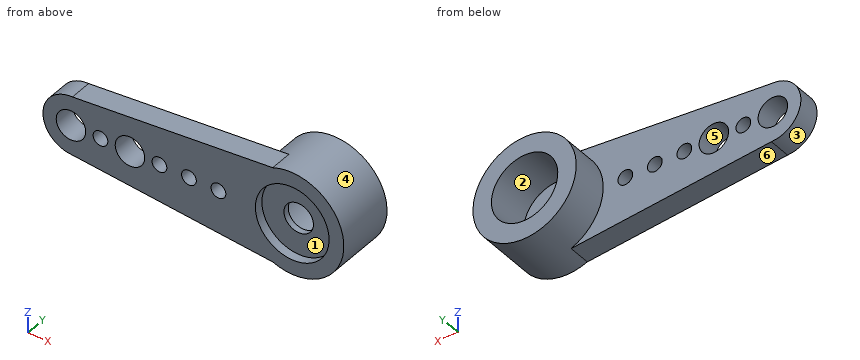
```python
from build123d import *

# Parameters (mm, degrees)
SKETCH1_R           = 3.5
BOSS_EXTRUDE1_DEPTH = 4
BOSS_EXTRUDE2_DEPTH = 1.5
SKETCH7_R           = 2.5
CUT_EXTRUDE4_DEPTH  = 0.6
SKETCH8_R           = 2.25
CUT_EXTRUDE5_DEPTH  = 3
SKETCH9_R           = 1
CUT_EXTRUDE6_DEPTH  = 18.590338257
SKETCH10_R          = 1
SKETCH10_R_2        = 0.5
CUT_EXTRUDE7_DEPTH  = 18.716094378


with BuildPart() as part:
    # Sketch1 → Boss-Extrude1 (new body)
    with BuildSketch(Plane(origin=(0, 0, 0), x_dir=(1, 0, 0), z_dir=(0, 1, 0))):
        with Locations(Location((0, 0, 0), (0, 0, 270))):
            Circle(SKETCH1_R)
    extrude(amount=BOSS_EXTRUDE1_DEPTH)

    # Sketch6 → Boss-Extrude2 (add)
    with BuildSketch(Plane.XZ):
        with BuildLine():
            Line((-14.9, 2), (-0.65, 3.301402389))
            Line((-0.65, 3.301402389), (0, 3.5))
            Line((0, 3.5), (0, -3.5))
            Line((0, -3.5), (-0.65, -3.301402389))
            Line((-0.65, -3.301402389), (-14.9, -2))
            ThreePointArc((-14.9, -2), (-16.9, 0), (-14.9, 2))
        make_face()
    extrude(amount=-BOSS_EXTRUDE2_DEPTH)

    # Sketch7 → Cut-Extrude4 (cut)
    with BuildSketch(Plane.XZ):
        with Locations(Location((0, 0, 0), (0, 0, 270))):
            Circle(SKETCH7_R)
    extrude(amount=-CUT_EXTRUDE4_DEPTH, mode=Mode.SUBTRACT)

    # Sketch8 → Cut-Extrude5 (cut)
    with BuildSketch(Plane(origin=(0, 4, 0), x_dir=(1, 0, 0), z_dir=(0, 1, 0))):
        with Locations(Location((0, 0, 0), (0, 0, 270))):
            Circle(SKETCH8_R)
    extrude(amount=-CUT_EXTRUDE5_DEPTH, mode=Mode.SUBTRACT)

    # Sketch9 → Cut-Extrude6 (cut, through all)
    with BuildSketch(Plane.XZ.offset(-0.6)):
        with Locations(Location((0, 0, 0), (0, 0, 270))):
            Circle(SKETCH9_R)
    extrude(amount=-CUT_EXTRUDE6_DEPTH, mode=Mode.SUBTRACT)

    # Sketch10 → Cut-Extrude7 (cut, through all)
    with BuildSketch(Plane.XZ):
        with Locations(Location((-15, 0, 0), (0, 0, 270))):
            Circle(SKETCH10_R)
        with Locations(Location((-13, 0, 0), (0, 0, 270))):
            Circle(SKETCH10_R_2)
        with Locations(Location((-11, 0, 0), (0, 0, 270))):
            Circle(SKETCH10_R)
        with Locations(Location((-9, 0, 0), (0, 0, 270))):
            Circle(SKETCH10_R_2)
        with Locations(Location((-7, 0, 0), (0, 0, 270))):
            Circle(SKETCH10_R_2)
        with Locations(Location((-5, 0, 0), (0, 0, 270))):
            Circle(SKETCH10_R_2)
    extrude(amount=-CUT_EXTRUDE7_DEPTH, mode=Mode.SUBTRACT)


solid = part.part
```
Here's how the part is built. I have some questions about the finished solid (model axes, mm). Face numbers are marked on the shaded views. A direction names the side the tool comes from. Give positions to 0.01 mm unless a question says otherwise; leave off trailing zeros. Write each loop counter-clockwise with the first axis right and the second up, starting at its lowest first coordinate (ties: lowest second). Pieces come first, ordered by that corner, then holes. Notation, with made-up numbers: (63.5, -19) -> (68.5, -19) arc R35 cw to (68.5, 14) -> close; hole circle Ø4 at (-39.5, -7). An arc over 180 degrees is marked (long way). Write each question's results on one line, items separated by ' | '.
Item 1: For pin 1 Ø1.5 at (x, y) = (-9.5, 1) entering from -Z; pin 2 Ø2 at (x, y) = (-2, 2.5) entering from +Z; pin 3 Ø2.5 at (x, z) = (0, 0) entering from +Y, each with a flat end and sliding along its axis, tell me the tip position at first contact or that it passes through.
Output:
pin 1: stops at z = -2.56 | pin 2: stops at z = 3.35 | pin 3: stops at y = 1
Item 2: Suppose I cut it at B-B on y = 1.3. Write out the boundary of the cut face in (x, z), plus the area to 3 significant figures.
Output:
outline: (-14.9, -2) -> (-1.32, -3.24) arc R3.5 ccw (long way) to (-1.32, 3.24) -> (-14.9, 2) arc R2 ccw to start; hole circle Ø2 at (-15, 0); hole circle Ø1 at (-13, 0); hole circle Ø2 at (-11, 0); hole circle Ø1 at (-9, 0); hole circle Ø1 at (-7, 0); hole circle Ø1 at (-5, 0); hole circle Ø4.5 at (0, 0) | area: 80.4 mm^2
Item 3: We'd pull the mould along X, two halves only. Please class the marked faces 4, 5 and 6: pulls with the +X half, pulls with the -X half, needs draft (parallel to the pull), parting line crosses it, or undercut.
Output:
face 4: parting line crosses it | face 5: undercut | face 6: pulls with the -X half
Item 4: Suppose I cut it at D-D on y = 3.75. Write out the boundary of the cut face in (x, z), plus the area to 3 significant figures.
Output:
outline: circle Ø7 at (0, 0); hole circle Ø4.5 at (0, 0) | area: 22.6 mm^2
Item 5: Suppose I cut it at C-C on z = 0.75. Write out the boundary of the cut face in (x, y).
Output:
outline: (-16.75, 0) -> (-15.66, 0) -> (-15.66, 1.5) -> (-16.75, 1.5) -> close; (-14.34, 0) -> (-11.66, 0) -> (-11.66, 1.5) -> (-14.34, 1.5) -> close; (-10.34, 0) -> (-2.38, 0) -> (-2.38, 0.6) -> (-0.66, 0.6) -> (-0.66, 1) -> (-2.12, 1) -> (-2.12, 4) -> (-3.42, 4) -> (-3.42, 1.5) -> (-10.34, 1.5) -> close; (0.66, 0.6) -> (2.38, 0.6) -> (2.38, 0) -> (3.42, 0) -> (3.42, 4) -> (2.12, 4) -> (2.12, 1) -> (0.66, 1) -> close
Item 6: Suppose I cut it at A-A on x = -5.25. Write out the boundary of the cut face in (y, z).
Output:
outline: (0, -2.88) -> (1.5, -2.88) -> (1.5, -0.43) -> (0, -0.43) -> close; (0, 0.43) -> (1.5, 0.43) -> (1.5, 2.88) -> (0, 2.88) -> close
Item 7: On a 3-axis mill with a long thin cutter (end or side, diameter ignored), from which of +Z, -Z, +X, -X, +Y, -Y can I reach the whole of each face in a straight line? I mean the marked faces 1, 2 and 3. Say none if no direction works.
Output:
face 1: -Y | face 2: +Y | face 3: -X, +Y, -Y
Item 8: If I drill on L1, parallel to X at y = 2.95, z = 0; L2, parallel to Y at x = -14, z = -1.5; L3, parallel to X at y = 3.45, z = -1.5, over which ranges is the centre line in solid material (lowest first)?
Output:
L1: x = -3.5 to -2.25, 2.25 to 3.5 | L2: y = 0 to 1.5 | L3: x = -3.16 to -1.68, 1.68 to 3.16
